Here's how the part is built. I have some questions about the finished solid (model axes, mm). A direction names the side the tool comes from. Coordinates: 2 decimals unless noted, no trailing zeros. Write each loop counter-clockwise with the first axis right and the second up, starting at its lowest first coordinate (ties: lowest second). Pieces come first, ordered by that corner, then holes. Notation, with made-up numbers: (66.5, 8) -> (76.5, 8) arc R21 cw to (76.5, 23) -> close; hole circle Ø3 at (-4.75, 49). An arc over 180 degrees is marked (long way). Use a Markdown table: item, result. Add a question column.
```python
from build123d import *

# Parameters (mm, degrees)
SKETCH1_R                = 2.1
BOSS_EXTRUDE1_DEPTH      = 17
BOSS_EXTRUDE1_DEPTH_BACK = 17
SKETCH2_R                = 2.75
CUT_EXTRUDE1_DEPTH       = 9
SKETCH3_R                = 2.75
CUT_EXTRUDE2_DEPTH       = 9


with BuildPart() as part:
    # Sketch1 → Boss-Extrude1 (new body, two sides)
    with BuildSketch(Plane(origin=(0, 0, 0), x_dir=(0, 0, -1), z_dir=(1, 0, 0))) as boss_extrude1_sk:
        Polygon((-70, 0), (0, 0), (49.497474683, 49.497474683), (43.133513652, 55.861435714), (28.991378029, 41.71930009), (-50, 9), (-70, 9), align=None)
        with Locations((-4.970562748, 12)):
            Circle(SKETCH1_R, mode=Mode.SUBTRACT)
        with BuildLine():
            Line((-6.551793043, 21.043679481), (-5.264121815, 17.934966139))
            ThreePointArc((-5.264121815, 17.934966139), (-4.812340099, 17.335290392), (-4.126543478, 17.029675086))
            ThreePointArc((-4.126543478, 17.029675086), (-0.768310337, 14.889822601), (0.028067769, 10.988222878))
            ThreePointArc((0.028067769, 10.988222878), (0.788934633, 9.368950353), (2.558913388, 9.6299812))
            Line((2.558913388, 9.6299812), (25.924897249, 32.995965061))
            ThreePointArc((25.924897249, 32.995965061), (26.111441495, 34.889980582), (24.290211928, 35.442444531))
            Line((24.290211928, 35.442444531), (-5.739998892, 23.003523928))
            ThreePointArc((-5.739998892, 23.003523928), (-6.551793043, 22.191729778), (-6.551793043, 21.043679481))
        make_face(mode=Mode.SUBTRACT)
        with BuildLine():
            Line((-41.663341292, 5), (-8.618850018, 5))
            ThreePointArc((-8.618850018, 5), (-7.182709356, 6.066987298), (-7.78969382, 7.75))
            ThreePointArc((-7.78969382, 7.75), (-9.985417083, 11.071971981), (-9.123891859, 14.959705611))
            ThreePointArc((-9.123891859, 14.959705611), (-8.855063072, 15.660739707), (-8.959639945, 16.40423241))
            Line((-8.959639945, 16.40423241), (-10.247311173, 19.512945751))
            ThreePointArc((-10.247311173, 19.512945751), (-11.059105323, 20.324739902), (-12.20715562, 20.324739902))
            Line((-12.20715562, 20.324739902), (-42.237366441, 7.885819299))
            ThreePointArc((-42.237366441, 7.885819299), (-43.134519213, 6.207364517), (-41.663341292, 5))
        make_face(mode=Mode.SUBTRACT)
    extrude(amount=BOSS_EXTRUDE1_DEPTH)
    extrude(boss_extrude1_sk.sketch, amount=-BOSS_EXTRUDE1_DEPTH_BACK)

    # Sketch2 → Cut-Extrude1 (cut)
    with BuildSketch(Plane(origin=(0, 0, 0), x_dir=(-1, 0, 0), z_dir=(0, 1, 0))):
        with Locations((10, 60)):
            Circle(SKETCH2_R)
    extrude(amount=CUT_EXTRUDE1_DEPTH, mode=Mode.SUBTRACT)

    # Sketch3 → Cut-Extrude2 (cut)
    with BuildSketch(Plane(origin=(0, 0, 0), x_dir=(-1, 0, 0), z_dir=(0, 1, 0))):
        with Locations((-10, 60)):
            Circle(SKETCH3_R)
    extrude(amount=CUT_EXTRUDE2_DEPTH, mode=Mode.SUBTRACT)

    # Sketch4 → Cut-Revolve1 (revolve, cut)
    with BuildSketch(Plane(origin=(10, 0, 0), x_dir=(0, 0, -1), z_dir=(1, 0, 0))):
        Polygon((-25, 30), (-20.5, 30), (-20.5, 9), (-22.25, 9), (-22.25, 0), (-25, 0), align=None)
    revolve(axis=Axis((10, 0, 25), (0, 1, 0)), mode=Mode.SUBTRACT)

    # Sketch5 → Cut-Revolve2 (revolve, cut)
    with BuildSketch(Plane(origin=(10, 0, 0), x_dir=(0, 0, -1), z_dir=(1, 0, 0))):
        Polygon((17.67766953, 17.67766953), (15.733125881, 15.733125881), (9.369164851, 22.097086912), (8.131727984, 20.859650045), (-6.717514421, 35.70889245), (-3.535533906, 38.890872965), align=None)
    revolve(axis=Axis((10, 38.890872965, 3.535533906), (0, -0.707106781, -0.707106781)), mode=Mode.SUBTRACT)

    # Sketch6 → Cut-Revolve3 (revolve, cut)
    with BuildSketch(Plane(origin=(-10, 0, 0), x_dir=(0, 0, -1), z_dir=(1, 0, 0))):
        Polygon((-25, 30), (-20.5, 30), (-20.5, 9), (-22.25, 9), (-22.25, 0), (-25, 0), align=None)
    revolve(axis=Axis((-10, 0, 25), (0, 1, 0)), mode=Mode.SUBTRACT)

    # Sketch7 → Cut-Revolve4 (revolve, cut)
    with BuildSketch(Plane(origin=(-10, 0, 0), x_dir=(0, 0, -1), z_dir=(1, 0, 0))):
        Polygon((17.67766953, 17.67766953), (15.733125881, 15.733125881), (9.369164851, 22.097086912), (8.131727984, 20.859650045), (-6.717514421, 35.70889245), (-3.535533906, 38.890872965), align=None)
    revolve(axis=Axis((-10, 38.890872965, 3.535533906), (0, -0.707106781, -0.707106781)), mode=Mode.SUBTRACT)

    # Sketch8 → Cut-Revolve5 (revolve, cut)
    with BuildSketch(Plane(origin=(10, 0, 0), x_dir=(0, 0, -1), z_dir=(1, 0, 0))):
        Polygon((36.062445841, 48.790367902), (38.006989489, 50.73491155), (44.370950519, 44.370950519), (42.426406871, 42.426406871), align=None)
    revolve(axis=Axis((10, 42.426406871, -42.426406871), (0, 0.707106781, 0.707106781)), mode=Mode.SUBTRACT)

    # Sketch9 → Cut-Revolve6 (revolve, cut)
    with BuildSketch(Plane(origin=(-10, 0, 0), x_dir=(0, 0, -1), z_dir=(1, 0, 0))):
        Polygon((36.062445841, 48.790367902), (38.006989489, 50.73491155), (44.370950519, 44.370950519), (42.426406871, 42.426406871), align=None)
    revolve(axis=Axis((-10, 42.426406871, -42.426406871), (0, 0.707106781, 0.707106781)), mode=Mode.SUBTRACT)


solid = part.part
```
Q1. Which directions (+Z, -Z, +X, -X, +Y, -Y) give clear straight access to the entire face, cutting with the end or side of a thin tool? Please do faces 5 (the cylindrical face through (0.24, 6.04, 7.19)), 6 (the cylindrical face through (8.648, 17.045, 20.708)), 7 (the flat face through (0, 9, 60)), 8 (the flat face through (0, 5, 70)), 9 (the flat face through (0, 24, -24)).
Q2. Suppose I cut it at C-C, the plane x = -3. Write out the boundary of the cut face in (y, z).
Q3. Suppose I cut it at D-D, the plane x = -10. State how many separate pieces and enclosed holes the cut face has, and give its area (3 significant figures).
Q4. Suppose I cut it at B-B, the plane y = 24.5. Write out the boundary of the cut face in (x, z), and give its area (3 significant figures).
Q5. Please list where these lines run through material, in increasing order: line 1 (X direction, y = 15.25, z = 25); line 2 (X direction, y = 2.4, z = 25); line 3 (Z direction, x = 10, y = 3).
Q6. Suppose I cut it at A-A, the plane z = 25. Write out the boundary of the cut face in (x, y), and give its area (3 significant figures).
Q7. Will these pins go through, and if not, where does the flat tip stop? pin 1 (4 mm diameter, centred on y = 12, z = 4.97, fed in from +X); pin 2 (10 mm diameter, centred on x = 4, z = 26, fed in from +Y); pin 3 (3 mm diameter, centred on x = -1.5, z = -31.5, fed in from -Y); pin 4 (14.5 mm diameter, centred on x = -10, z = 25, fed in from +Y).
Q8. Thinking about a two-plate mould opening in Z: for faces 1 (the cylindrical face through (8.648, 26.777, -2.508)), 2 (the cylindrical face through (-9.642, 4.437, 62.727)), 3 (the flat face through (0.24, 48.89, -36.16)), 4 (the flat face through (0.238, 52.635, -46.36)), which applies, released by +Z, released by -Z, zero draft, split by the parting line, or undercut?
Answer key:
| question | item | result |
|---|---|---|
| 1 | face 5 | +X, -X |
| 1 | face 6 | +Y |
| 1 | face 7 | +Z, +X, -X, +Y |
| 1 | face 8 | +Z, +X, -X, +Y, -Y |
| 1 | face 9 | -Z, +X, -X, -Y |
| 2 | outline | (0, 0) -> (49.5, -49.5) -> (55.86, -43.13) -> (41.72, -28.99) -> (9, 50) -> (9, 70) -> (0, 70) -> close; hole (5, 8.62) arc R1.5 ccw to (7.75, 7.79) arc R5.1 cw to (14.96, 9.12) arc R1.5 ccw to (16.4, 8.96) -> (19.51, 10.25) arc R1.5 ccw to (20.32, 12.21) -> (7.89, 42.24) arc R1.5 ccw to (5, 41.66) -> close; hole (9.63, -2.56) -> (33, -25.92) arc R1.5 ccw to (35.44, -24.29) -> (23, 5.74) arc R1.5 ccw to (21.04, 6.55) -> (17.93, 5.26) arc R1.5 ccw to (17.03, 4.13) arc R5.1 cw to (10.99, -0.03) arc R1.5 ccw to start; hole circle Ø4.2 at (12, 4.97) |
| 3 | separate pieces | 5 |
| 3 | enclosed holes | 1 |
| 3 | area | 1,090 mm^2 |
| 4 | outline | (-17, -24.5) -> (17, -24.5) -> (17, -17.43) -> (-17, -17.43) -> close; (-17, 2.13) -> (17, 2.13) -> (17, 12.58) -> (-17, 12.58) -> close |
| 4 | area | 596 mm^2 |
| 5 | line 1 | x = -17 to -14.5, -5.5 to 5.5, 14.5 to 17 |
| 5 | line 2 | x = -17 to -12.75, -7.25 to 7.25, 12.75 to 17 |
| 5 | line 3 | z = -3 to 22.25, 27.75 to 57.25, 62.75 to 70 |
| 6 | outline | (-17, 0) -> (-12.75, 0) -> (-12.75, 5) -> (-17, 5) -> close; (-17, 15.03) -> (-14.5, 15.03) -> (-14.5, 19.36) -> (-17, 19.36) -> close; (-7.25, 0) -> (7.25, 0) -> (7.25, 5) -> (-7.25, 5) -> close; (-5.5, 15.03) -> (5.5, 15.03) -> (5.5, 19.36) -> (-5.5, 19.36) -> close; (12.75, 0) -> (17, 0) -> (17, 5) -> (12.75, 5) -> close; (14.5, 15.03) -> (17, 15.03) -> (17, 19.36) -> (14.5, 19.36) -> close |
| 6 | area | 184 mm^2 |
| 7 | pin 1 | passes through |
| 7 | pin 2 | stops at y = 21.01 |
| 7 | pin 3 | stops at y = 30 |
| 7 | pin 4 | stops at y = 22.36 |
| 8 | face 1 | undercut |
| 8 | face 2 | undercut |
| 8 | face 3 | released by +Z |
| 8 | face 4 | released by -Z |
